CAD build for the part. Positions are in the model's coordinates, mm. Face numbers are marked on the shaded views. A direction names the side the tool comes from. Round coordinates to 2 decimals unless told otherwise and drop trailing zeros. Write each loop counter-clockwise with the first axis right and the second up, starting at its lowest first coordinate (ties: lowest second). Pieces come first, ordered by that corner, then holes. Notation, with made-up numbers: (-12, 32.25) - (16, 32.25) arc R19 ccw to (16, 58.25) - close; hole circle Ø10 at (24.25, 5.25). An arc over 180 degrees is marked (long way). Use one line per item in the form item = value. Start each with the question number.
Item 1: Band-saw the part on C-C, the plane x = 43.5. List the corners of the cut face in (y, z), and give its area (3 significant figures).
Item 2: Drill centre lines: L1, parallel to Z at x = 3.5, y = 122; L2, parallel to Y at x = 157.5, z = 290.5; L3, parallel to Z at x = -15, y = -117.5. Where is each one in solid material? Low to high.
Item 3: Tool access for the marked faces 1, 2, 3 and 4: list every direction of +Z, -Z, +X, -X, +Y, -Y with a clear straight run to the whole face (end or side of a thin tool).
Item 4: Pin check, flat tips, straight feed: pin 1 (1.5 mm diameter, centred on x = 153.5, y = 153.5, fed in from +Z); pin 2 (1 mm diameter, centred on x = 22.5, y = 402, fed in from +Z). Stop position of each tip, or through.
Item 5: Band-saw the part on A-A, the plane x = 160. List the corners of the cut face in (y, z), and give its area (3 significant figures).
Item 6: Band-saw the part on B-B, the plane y = 86. List the corners of the cut face in (x, z).
Item 7: Band-saw the part on D-D, the plane y = 168.5. List the corners of the cut face in (x, z).
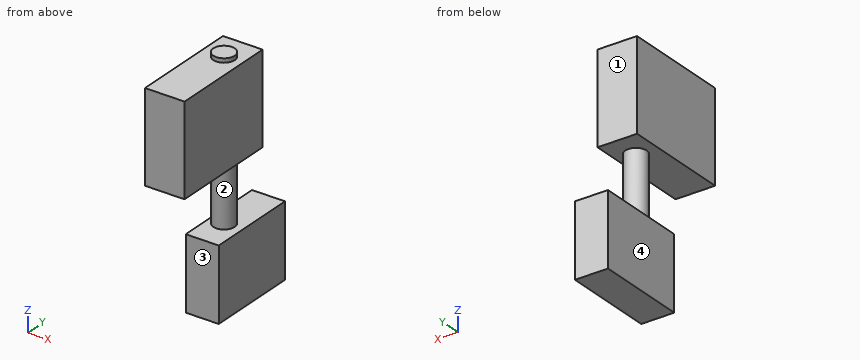
from build123d import *

# Parameters (mm, degrees)
F0_W     = 190.5
F0_H     = 533.4
F1_DEPTH = 419.1
F2_R     = 61.948807
F3_DEPTH = 914.4
F4_W     = 627.843589
F4_H     = 522.065521
F5_DEPTH = 228.6


with BuildPart() as f1:
    # F0 (on Top) → F1 (new body)
    with BuildSketch(Plane.XY):
        with Locations((95.25, 266.7)):
            Rectangle(F0_W, F0_H)
    extrude(amount=F1_DEPTH)

    # F2 (on face) → F3 (join)
    with BuildSketch(Plane.XY.offset(419.1)):
        with Locations((82.928531, 192.244217)):
            Circle(F2_R)
    extrude(amount=F3_DEPTH)

    # F4 (on face) → F5 (join)
    with BuildSketch(Plane.YZ.offset(190.5)):
        with Locations((38.371071, 1048.732937)):
            Rectangle(F4_W, F4_H)
    extrude(amount=-F5_DEPTH)


solid = f1.part
Determined:
q1.outline = (-275.55, 787.7) - (144.46, 787.7) - (144.46, 419.1) - (0, 419.1) - (0, 0) - (533.4, 0) - (533.4, 419.1) - (240.03, 419.1) - (240.03, 787.7) - (352.29, 787.7) - (352.29, 1309.77) - (240.03, 1309.77) - (240.03, 1333.5) - (144.46, 1333.5) - (144.46, 1309.77) - (-275.55, 1309.77) - close
q1.area = 589,000 mm²
q2.L1 = 0 to 419.1, 787.7 to 1309.77
q2.L2 = 0 to 533.4
q2.L3 = 787.7 to 1309.77
q3.face_1 = +Z, +X, -X, +Y
q3.face_2 = none
q3.face_3 = -Z, +X, -X, -Y
q3.face_4 = -Z, -X, +Y, -Y
q4.pin_1 = 1309.77
q4.pin_2 = 419.1
q5.outline = (-275.55, 787.7) - (352.29, 787.7) - (352.29, 1309.77) - (-275.55, 1309.77) - close; (0, 0) - (533.4, 0) - (533.4, 419.1) - (0, 419.1) - close
q5.area = 551,000 mm²
q6.outline = (-38.1, 787.7) - (190.5, 787.7) - (190.5, 1309.77) - (-38.1, 1309.77) - close; (0, 0) - (190.5, 0) - (190.5, 419.1) - (0, 419.1) - close
q7.outline = (-38.1, 787.7) - (25.71, 787.7) - (25.71, 419.1) - (0, 419.1) - (0, 0) - (190.5, 0) - (190.5, 419.1) - (140.15, 419.1) - (140.15, 787.7) - (190.5, 787.7) - (190.5, 1309.77) - (140.15, 1309.77) - (140.15, 1333.5) - (25.71, 1333.5) - (25.71, 1309.77) - (-38.1, 1309.77) - close
